Geometry check sheet. Reference: drawing and pictorial views, mm from the part's lowest x, y, z. A direction names the side the tool comes from. Coordinates: 2 decimals unless noted, no trailing zeros. Write each loop counter-clockwise with the first axis right and the second up, starting at its lowest first coordinate (ties: lowest second). Pieces come first, ordered by that corner, then holes. Notation, with made-up numbers: (67.5, 67) -> (83.5, 67) arc R29 ccw to (83.5, 99) -> close; hole circle Ø3 at (2.5, 87.25). An arc over 180 degrees is marked (long way). Use a Markdown table: item, result.
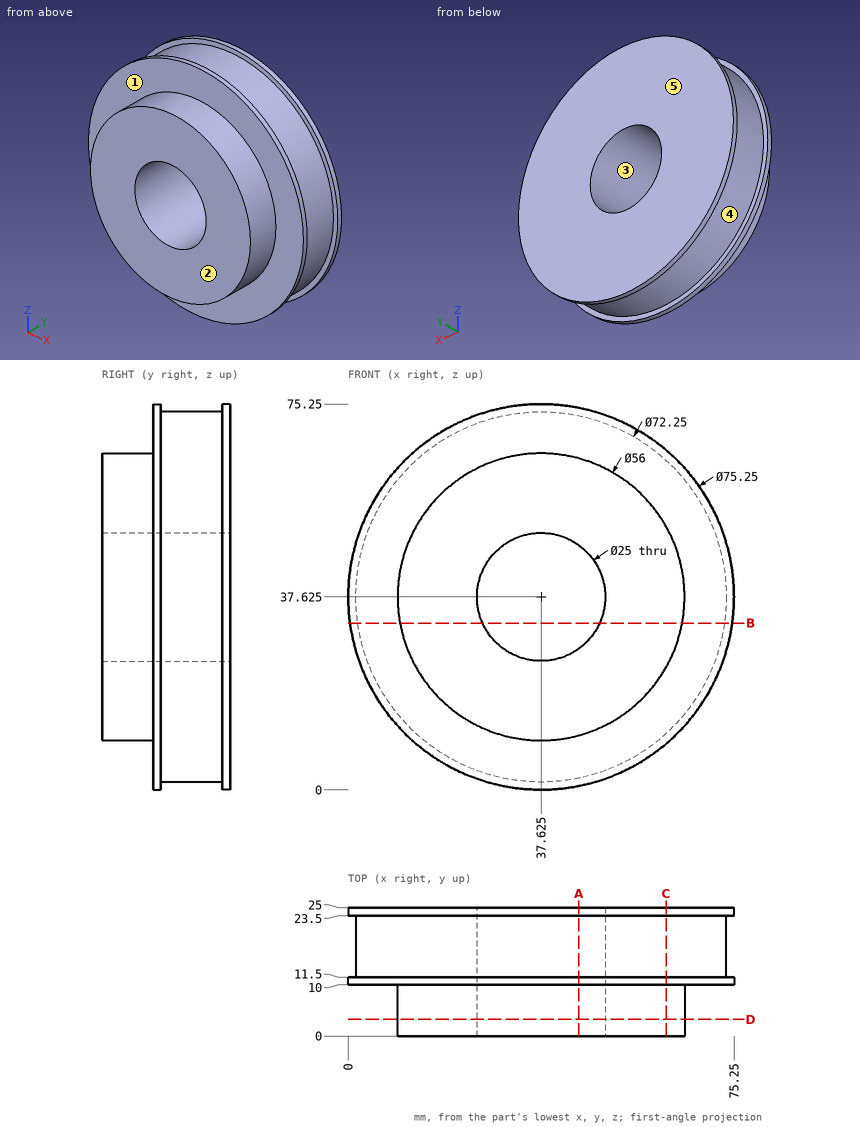
Item 1: Mould release check, pull along Y, two halves, no side actions. Record for the marked faces 3, 4 and 5: +Y half, -Y half, draft (parallel to the pull), parting line (faces both ways), or undercut.
Answer block:
| item | result |
|---|---|
| face 3 | draft |
| face 4 | undercut |
| face 5 | +Y half |
Item 2: Section check D-D on y = 3.25. Record the boundary of the cut face in (x, z) (3 decimals).
Answer block:
| item | result |
|---|---|
| outline | circle Ø56 at (37.625, 37.625); hole circle Ø25 at (37.625, 37.625) |
Item 3: Section check B-B on z = 32.5. Record the boundary of the cut face in (x, y).
Answer block:
| item | result |
|---|---|
| outline | (0.35, 10) -> (10.1, 10) -> (10.1, 0) -> (26.22, 0) -> (26.22, 25) -> (0.35, 25) -> (0.35, 23.5) -> (1.87, 23.5) -> (1.87, 11.5) -> (0.35, 11.5) -> close; (49.03, 0) -> (65.15, 0) -> (65.15, 10) -> (74.9, 10) -> (74.9, 11.5) -> (73.38, 11.5) -> (73.38, 23.5) -> (74.9, 23.5) -> (74.9, 25) -> (49.03, 25) -> close |
Item 4: Depth check by flat-ended pin: P1, Ø10, axis at y = 12.5, z = 59.5, coming from the -X side; P2, Ø1.5, axis at x = 30.5, y = 6, coming from the -Z side; P3, Ø6, axis at x = 18.5, y = 17.5, coming from the +Z side. Enter the tip coordinate at first touch or a pass-through.
Answer block:
| item | result |
|---|---|
| P1 | stops at x = 4.05 |
| P2 | stops at z = 10.36 |
| P3 | stops at z = 69.95 |
Item 5: Section check A-A on x = 45. Record the boundary of the cut face in (y, z), then the cut area to 3 significant figures.
Answer block:
| item | result |
|---|---|
| outline | (0, 10.61) -> (10, 10.61) -> (10, 0.73) -> (11.5, 0.73) -> (11.5, 2.26) -> (23.5, 2.26) -> (23.5, 0.73) -> (25, 0.73) -> (25, 27.53) -> (0, 27.53) -> close; (0, 47.72) -> (25, 47.72) -> (25, 74.52) -> (23.5, 74.52) -> (23.5, 72.99) -> (11.5, 72.99) -> (11.5, 74.52) -> (10, 74.52) -> (10, 64.64) -> (0, 64.64) -> close |
| area | 1,110 mm^2 |
Item 6: Tool access check on the marked faces 1 and 2. Record the directions out of +Z, -Z, +X, -X, +Y, -Y that give a thin tool (end or side, any length) a straight path to the whole face; none if there is none.
Answer block:
| item | result |
|---|---|
| face 1 | -Y |
| face 2 | +Z, -Z, +X, -X, -Y |
Item 7: Section check C-C on x = 62. Record the boundary of the cut face in (y, z), then the cut area to 3 significant figures.
Answer block:
| item | result |
|---|---|
| outline | (0, 23.85) -> (10, 23.85) -> (10, 8.96) -> (11.5, 8.96) -> (11.5, 10.96) -> (23.5, 10.96) -> (23.5, 8.96) -> (25, 8.96) -> (25, 66.29) -> (23.5, 66.29) -> (23.5, 64.29) -> (11.5, 64.29) -> (11.5, 66.29) -> (10, 66.29) -> (10, 51.4) -> (0, 51.4) -> close |
| area | 1,090 mm^2 |
Item 8: Thickness scan on L1, parallel to Y at x = 51, z = 11; L2, parallel to X at y = 3, z = 33; L3, parallel to Z at x = 45, y = 6.75. Record the ranges inside material, lowest first. Write a range as [from, to].
Answer block:
| item | result |
|---|---|
| L1 | y = [10, 25] |
| L2 | x = [10.01, 26.01], [49.24, 65.24] |
| L3 | z = [10.61, 27.53], [47.72, 64.64] |
